Build history of the part. All positions in model axes, mm. A direction names the side the tool comes from. Coordinates: 2 decimals unless noted, no trailing zeros. Write each loop counter-clockwise with the first axis right and the second up, starting at its lowest first coordinate (ties: lowest second). Pieces come first, ordered by that corner, then holes.
from build123d import *

# Parameters (mm, degrees)
F0_R     = 6.35
F1_DEPTH = 22.86
F2_DEPTH = 3.175
F3_ANGLE = 180


with BuildPart() as f1:
    # F0 (on Top) → F1 (new body)
    with BuildSketch(Plane.XY):
        with Locations((-4.509694, 23.622)):
            Circle(F0_R)
    extrude(amount=-F1_DEPTH)

    # F0 (on Top) → F2 (join)
    with BuildSketch(Plane.XY):
        with BuildLine():
            Line((0, 57.15), (-25.4, 57.15))
            Line((-25.4, 57.15), (-25.4, 34.925))
            ThreePointArc((-25.4, 34.925), (-15.170704, 10.229296), (9.525, 0))
            Line((9.525, 0), (19.05, 0))
            Line((19.05, 0), (69.85, 0))
            Line((69.85, 0), (69.85, 25.4))
            Line((69.85, 25.4), (19.05, 25.4))
            Line((19.05, 25.4), (9.525, 25.4))
            ThreePointArc((9.525, 25.4), (2.789808, 28.189808), (0, 34.925))
            Line((0, 34.925), (0, 57.15))
        make_face()
        with Locations((-4.509694, 23.622)):
            Circle(F0_R, mode=Mode.SUBTRACT)
    extrude(amount=-F2_DEPTH)


with BuildPart() as f1_1:
    # F3: moved
    add(f1.part.rotate(Axis((0, 46.0375, -3.175), (0, 1, 0)), F3_ANGLE))


solid = f1_1.part
(1) Slice it at B-B, the plane x = 9. List the corners of the cut face in (y, z) (3 decimals), and give its area (3 significant figures).
(2) 3-axis set-ups, long thin cutter, end or side, ignore diameter. For faces 1 (the flat face through (-39, 0, -5)), 2 (the cylindrical face through (-1.356, 21.19, 6.53)), 3 (the flat face through (0, 46, -5)): which of +Z, -Z, +X, -X, +Y, -Y reach the whole face in a straight line?
(3) Probe L1, parallel to Y at x = 4, z = 0.75; L2, parallel to X at y = 45, z = -5; L3, parallel to Z at x = -62, y = 21 (3 decimals). List the from-to ranges inside material, lowest first.
(4) Flat gauge pins, fed straight in: P1, Ø17, axis at x = -9, y = 40.5, coming from the +Z side; P2, Ø12, axis at y = 16.5, z = -4, coming from the +X side; P3, Ø1.6, axis at x = -29.5, z = -4.5, coming from the +Y side; P4, Ø1, axis at y = 43.5, z = -5.5, coming from the -X side. Where does each tip first touch, or does it go through?
(5) Slice it at A-A, the plane y = 52. List the corners of the cut face in (x, z) (3 decimals), and give its area (3 significant figures).
(6) Slice it at C-C, the plane z = 7. List the corners of the cut face in (x, y), and give its area (3 significant figures).
(7) Slice it at D-D, the plane y = 22. List the corners of the cut face in (x, z) (3 decimals), and give its area (3 significant figures).
Results:
1. outline: (5.318, -6.35) - (57.15, -6.35) - (57.15, -3.175) - (28.112, -3.175) - (28.112, 16.51) - (19.132, 16.51) - (19.132, -3.175) - (5.318, -3.175) - close
1. area: 341 mm2
2. face 1: +Z, -Z, +X, -X, -Y
2. face 2: +Z
2. face 3: +Z, -Z, -X, +Y
3. L1: y = 17.29 to 29.95
3. L2: x = 0 to 25.4
3. L3: z = -6.35 to -3.175
4. P1: passes through
4. P2: stops at x = 23.12
4. P3: stops at y = 25.4
4. P4: stops at x = 0
5. outline: (0, -6.35) - (25.4, -6.35) - (25.4, -3.175) - (0, -3.175) - close
5. area: 80.6 mm2
6. outline: circle Ø12.7 at (4.51, 23.62)
6. area: 127 mm2
7. outline: (-69.85, -6.35) - (22.92, -6.35) - (22.92, -3.175) - (10.649, -3.175) - (10.649, 16.51) - (-1.63, 16.51) - (-1.63, -3.175) - (-69.85, -3.175) - close
7. area: 536 mm2
